CAD build for the part. Positions are in the model's coordinates, mm. A direction names the side the tool comes from. Give positions to 0.01 mm unless a question says otherwise; leave off trailing zeros. Loops run counter-clockwise (first coordinate to the right, second up) from the corner with the lowest first, then second, coordinate; pieces in that order, holes last. Notation, with made-up numbers: (76.25, -26.75) -> (132.25, -26.75) arc R29 cw to (132.25, 0.25) -> close; hole circle Ø11 at (20, -15.75). An arc over 180 degrees is marked (long way). Use one line per item in the form item = value.
Autodesk Inventor part; units mm, degrees
ref_plane "YZ Plane" through (0, 0, 0) normal (1, 0, 0) x (0, 1, 0)
ref_plane "XZ Plane" through (0, 0, 0) normal (0, 1, 0) x (-1, 0, 0)
ref_plane "XY Plane" through (0, 0, 0) normal (0, 0, 1) x (1, 0, 0)
sketch "Эскиз1" plane through (0, 0, 0) normal (0, 0, 1) x (1, 0, 0)
  circle A0 centre (0, 0) radius 7.6
  circle A1 centre (0, 0) radius 11.5
  line L0 (8.8095, 7.3921) -> (0, 0)
  line L1 (-16.1, 0) -> (16.1, 0) construction
  line L2 (0, 0) -> (-10.8065, 3.9332)
  line L3 (8.8095, 7.3921) -> (11.5, 7.3921)
  line L4 (11.5, 7.3921) -> (11.5, -11.5)
  line L5 (11.5, -11.5) -> (0, -11.5)
  point P0 (5.8219, 4.8852)
  point P1 (-5.8219, -4.8852)
  point P2 (-7.1417, 2.5994)
  point P3 (11.5, 0)
  dimension "d0" = 15.2
  dimension "d2" = 23
  dimension "d8" = 40
  dimension "d11" = 20
extrude "Выдавливание1" add sketch "Эскиз1" along normal blind 8 contours A0 L0 A1 L2 | L3 L4 A1 | L4 L5 A1 picked at (-9.7933, 2.5948)
sketch "Эскиз2" plane through (0, 0, 0) normal (1, 0, 0) x (0, 1, 0)
  circle A0 centre (0, 4) radius 2.1
  line L0 (3.9332, 8) -> (-11.5, 8)
  line L1 (3.9332, 0) -> (-11.5, 0)
  line L2 (0, 8) -> (0, 0) construction
  dimension "d5" = 4.2
extrude "Выдавливание2" cut sketch "Эскиз2" along normal blind 15
fillet "Сопряжение1" radius 1.6 6 edges at (8.8095, 7.3921, 4) (5.8219, 4.8852, 4) (-7.1417, 2.5994, 4) (-10.8065, 3.9332, 4) (11.5, 7.3921, 4) (11.5, -11.5, 4)
fillet "Сопряжение1" radius 0.6 2 edges at (7.3041, -2.1, 4.0117) (11.5, -2.1, 4)
properties part number "Кольцо линейного подшипника"
1. Cut at C-C, the plane z = 7.75. Write the cut outline in (x, y), then the cut area to 3 significant figures.
Result sheet:
outline = (-11.3, 2.13) arc R11.5 ccw to (0, -11.5) -> (9.9, -11.5) arc R1.6 ccw to (11.5, -9.9) -> (11.5, 5.79) arc R1.6 ccw to (9.9, 7.39) -> (9.39, 7.39) arc R1.6 ccw to (8.36, 7.02) -> (6.94, 5.82) arc R1.6 ccw to (6.58, 3.8) arc R7.6 cw (long way) to (-7.48, 1.32) arc R1.6 ccw to (-8.51, 3.1) -> (-9.18, 3.34) arc R1.6 ccw to start
area = 188 mm^2
2. Drop a flat-ended pin along its axis: P1, Ø3, axis at x = -6, z = 6.5, coming from the -Y side. Give the stop position or say it passes through.
Result sheet:
P1 = -10.58
3. Mould opens along X. For faces 3 (the cylindrical face through (-10.5, 3.24, 4.06)), 4 (the cylindrical face through (6.396, 4.891, 4.056)), 5 (the flat face through (5, -6, 8)) say: pulls with the +X half, pulls with the -X half, needs draft (parallel to the pull), parting line crosses it, or undercut.
Result sheet:
face_3 = undercut
face_4 = pulls with the -X half
face_5 = needs draft
4. Cut at A-A, the plane y = -7. Write the cut outline in (x, z), then the cut area to 3 significant figures.
Result sheet:
outline = (-9.12, 0) -> (-2.96, 0) -> (-2.96, 8) -> (-9.12, 8) -> close; (2.96, 0) -> (11.5, 0) -> (11.5, 8) -> (2.96, 8) -> close
area = 118 mm^2
5. Drill centre lines: line 1 (Z direction, x = 10.35, y = 0); line 2 (Y direction, x = 9.8, z = 4); line 3 (Y direction, x = 0, z = 4). Where is each one in solid material? Low to high.
Result sheet:
line_1 = 0 to 1.9, 6.1 to 8
line_2 = -11.5 to -2.1, 2.1 to 7.39
line_3 = -11.5 to -7.6
6. Cut at B-B, the plane y = 0. State how many separate pieces and enclosed holes the cut face has, then the cut area to 3 significant figures.
Result sheet:
separate_pieces = 3
enclosed_holes = 0
area = 45.7 mm^2
7. Tool access for faces 1 (the cylindrical face through (9.3, 1.94, 4.8)), 2 (the flat face through (11.5, -4, 4)): list every direction of +Z, -Z, +X, -X, +Y, -Y with a clear straight run to the whole face (end or side of a thin tool).
Result sheet:
face_1 = +X
face_2 = +Z, -Z, +X, +Y, -Y
8. Cut at D-D, the plane x = -5.5. Write the cut outline in (y, z) (1 decimal), then the cut area to 3 significant figures.
Result sheet:
outline = (-10.1, 0) -> (-5.2, 0) -> (-5.2, 8) -> (-10.1, 8) -> close
area = 38.8 mm^2
